from build123d import *

# Parameters (mm, degrees)
SKETCH4_R           = 2
BOSS_EXTRUDE3_DEPTH = 6
SKETCH6_R           = 3.276903459
BOSS_EXTRUDE4_DEPTH = 6
CUT_EXTRUDE1_DEPTH  = 10


with BuildPart() as part:
    # Sketch4 → Boss-Extrude3 (new body)
    with BuildSketch(Plane.XY):
        with BuildLine():
            ThreePointArc((11.330682707, 3.9516616), (8.917819898, 4.428819506), (6.681915604, 3.403968986))
            ThreePointArc((6.681915604, 3.403968986), (6.066818441, 4.407801607), (5.302192362, 5.302995112))
            ThreePointArc((5.302192362, 5.302995112), (6.967815552, 7.112770233), (7.259627029, 9.554989032))
            ThreePointArc((7.259627029, 9.554989032), (7.053423028, 9.708203932), (6.843986457, 9.856969584))
            ThreePointArc((6.843986457, 9.856969584), (4.61147306, 8.824753264), (3.40498051, 6.681400208))
            ThreePointArc((3.40498051, 6.681400208), (2.317318441, 7.131972816), (1.172541409, 7.406763642))
            ThreePointArc((1.172541409, 7.406763642), (1.456299749, 9.849931218), (0.256880001, 11.997250213))
            ThreePointArc((0.256880001, 11.997250213), (0, 12), (-0.256880001, 11.997250213))
            ThreePointArc((-0.256880001, 11.997250213), (-1.456299749, 9.849931218), (-1.172541409, 7.406763642))
            ThreePointArc((-1.172541409, 7.406763642), (-2.317318441, 7.131972816), (-3.404980509, 6.681400207))
            ThreePointArc((-3.404980509, 6.681400207), (-4.61147306, 8.824753264), (-6.843986457, 9.856969584))
            ThreePointArc((-6.843986457, 9.856969584), (-7.053423028, 9.708203933), (-7.259627029, 9.554989032))
            ThreePointArc((-7.259627029, 9.554989032), (-6.967815552, 7.112770233), (-5.302192362, 5.302995112))
            ThreePointArc((-5.302192362, 5.302995112), (-6.066818441, 4.407801607), (-6.681915604, 3.403968986))
            ThreePointArc((-6.681915604, 3.403968986), (-8.917819898, 4.428819506), (-11.330682707, 3.9516616))
            ThreePointArc((-11.330682707, 3.9516616), (-11.412678196, 3.708203933), (-11.489443278, 3.463046803))
            ThreePointArc((-11.489443278, 3.463046803), (-9.817862641, 1.658772773), (-7.406586048, 1.173662691))
            ThreePointArc((-7.406586048, 1.173662691), (-7.499, 0), (-7.406586048, -1.173662691))
            ThreePointArc((-7.406586048, -1.173662691), (-9.817862641, -1.658772773), (-11.489443278, -3.463046803))
            ThreePointArc((-11.489443278, -3.463046803), (-11.412678196, -3.708203933), (-11.330682707, -3.9516616))
            ThreePointArc((-11.330682707, -3.9516616), (-8.917819898, -4.428819506), (-6.681915604, -3.403968986))
            ThreePointArc((-6.681915604, -3.403968986), (-6.066818441, -4.407801607), (-5.302192362, -5.302995112))
            ThreePointArc((-5.302192362, -5.302995112), (-6.967815552, -7.112770233), (-7.259627029, -9.554989032))
            ThreePointArc((-7.259627029, -9.554989032), (-7.053423028, -9.708203932), (-6.843986457, -9.856969584))
            ThreePointArc((-6.843986457, -9.856969584), (-4.61147306, -8.824753264), (-3.404980509, -6.681400207))
            ThreePointArc((-3.404980509, -6.681400207), (-2.317318441, -7.131972816), (-1.172541409, -7.406763642))
            ThreePointArc((-1.172541409, -7.406763642), (-1.456299749, -9.849931218), (-0.256880001, -11.997250213))
            ThreePointArc((-0.256880001, -11.997250213), (0, -12), (0.256880001, -11.997250213))
            ThreePointArc((0.256880001, -11.997250213), (1.456299749, -9.849931218), (1.172541409, -7.406763642))
            ThreePointArc((1.172541409, -7.406763642), (2.317318441, -7.131972816), (3.404980509, -6.681400207))
            ThreePointArc((3.404980509, -6.681400207), (4.61147306, -8.824753264), (6.843986457, -9.856969584))
            ThreePointArc((6.843986457, -9.856969584), (7.053423027, -9.708203933), (7.259627029, -9.554989032))
            ThreePointArc((7.259627029, -9.554989032), (6.967815552, -7.112770233), (5.302192362, -5.302995112))
            ThreePointArc((5.302192362, -5.302995112), (6.066818441, -4.407801607), (6.681915604, -3.403968986))
            ThreePointArc((6.681915604, -3.403968986), (8.917819898, -4.428819506), (11.330682707, -3.9516616))
            ThreePointArc((11.330682707, -3.9516616), (11.412678196, -3.708203932), (11.489443278, -3.463046803))
            ThreePointArc((11.489443278, -3.463046803), (9.817862641, -1.658772773), (7.406586048, -1.173662691))
            ThreePointArc((7.406586048, -1.173662691), (7.499, 0), (7.406586048, 1.173662691))
            ThreePointArc((7.406586048, 1.173662691), (9.817862641, 1.658772773), (11.489443278, 3.463046803))
            ThreePointArc((11.489443278, 3.463046803), (11.412678196, 3.708203932), (11.330682707, 3.9516616))
        make_face()
        Circle(SKETCH4_R, mode=Mode.SUBTRACT)
    extrude(amount=BOSS_EXTRUDE3_DEPTH)

    # Sketch6 → Boss-Extrude4 (add)
    with BuildSketch(Plane.XY.offset(6)):
        Circle(SKETCH6_R)
    extrude(amount=-BOSS_EXTRUDE4_DEPTH)

    # Sketch7 → Cut-Extrude1 (cut)
    with BuildSketch(Plane.XY.offset(6)):
        with BuildLine():
            Line((-1.288409873, 1.875), (1.288409873, 1.875))
            ThreePointArc((1.288409873, 1.875), (0, -2.275), (-1.288409873, 1.875))
        make_face()
    extrude(amount=-CUT_EXTRUDE1_DEPTH, mode=Mode.SUBTRACT)


solid = part.part
Source: CAD feature listing. Evaluate the final solid. Frame: model axes, mm. A direction names the side the tool comes from. Coordinates: 2 decimals unless noted, no trailing zeros. Order: outer loops, then holes, each group sorted by start corner. A loop starts at its lowest first (then second) coordinate and runs counter-clockwise, first axis right, second up.
Item 1: Cut plane A-A (y = 0). Return loops of the section in (x, z) (3 decimals), plus the area to 3 significant figures.
Output values:
outline: (-7.499, 0) - (-2.275, 0) - (-2.275, 6) - (-7.499, 6) - close; (2.275, 0) - (7.499, 0) - (7.499, 6) - (2.275, 6) - close
area: 62.7 mm2
Item 2: Cut plane B-B (x = 5.75). Return loops of the section in (y, z).
Output values:
outline: (-9.56, 0) - (-5.6, 0) - (-5.6, 6) - (-9.56, 6) - close; (-4.81, 0) - (4.81, 0) - (4.81, 6) - (-4.81, 6) - close; (5.6, 0) - (9.56, 0) - (9.56, 6) - (5.6, 6) - close
Item 3: Pull-direction query (X, two-part tool) for faces 1 (the face through (-3, 0, 6)), 2 (the face through (2.333, 7.127, 2.958)); classes: pulls with the +X half, pulls with the -X half, needs draft (parallel to the pull), parting line crosses it, or undercut.
Output values:
face 1: needs draft
face 2: undercut
Item 4: Material intervals for line 1 (X direction, y = 0, z = 1.3) (3 decimals); line 2 (X direction, y = 9.25, z = 2.05); line 3 (Y direction, x = 0, z = 1.8) (3 decimals), sorted ascending.
Output values:
line 1: x = -7.499 to -2.275, 2.275 to 7.499
line 2: x = -7.31 to -5.16, -1.53 to 1.53, 5.16 to 7.31
line 3: y = -12 to -2.275, 1.875 to 12
Item 5: Cut plane D-D (x = -9.5). Return loops of the section in (y, z), plus the area to 3 significant figures.
Output values:
outline: (-4.45, 0) - (-1.5, 0) - (-1.5, 6) - (-4.45, 6) - close; (1.5, 0) - (4.45, 0) - (4.45, 6) - (1.5, 6) - close
area: 35.5 mm2
Item 6: Set-up query: faces 3 (the face through (0, 1.875, 3)), 4 (the face through (-3, 0, 0)). Return all of +Z, -Z, +X, -X, +Y, -Y with unobstructed straight access to the full face (end or side cutting, diameter ignored); none if empty.
Output values:
face 3: +Z, -Z
face 4: -Z, +X, -X, +Y, -Y
Item 7: First-contact query: P1, Ø1.5, axis at x = 6.5, z = 2, coming from the +Y side; P2, Ø12, axis at x = -2, y = -4.5, coming from the -Z side. Flat tips, straight axial feed; report the tip coordinate or a pass-through.
Output values:
P1: stops at y = 9.86
P2: stops at z = 0
Item 8: Cut plane C-C (y = -9). Return loops of the section in (x, z), plus the area to 3 significant figures.
Output values:
outline: (-7.33, 0) - (-4.81, 0) - (-4.81, 6) - (-7.33, 6) - close; (-1.53, 0) - (1.53, 0) - (1.53, 6) - (-1.53, 6) - close; (4.81, 0) - (7.33, 0) - (7.33, 6) - (4.81, 6) - close
area: 48.6 mm2
